```python
from build123d import *

# Parameters (mm, degrees)
F0_R     = 2.38125
F0_R_2   = 1.143
F1_DEPTH = 4.7625
F2_R     = 6.35
F3_DEPTH = 7.62
F4_DEPTH = 5.08


with BuildPart() as f1:
    # F0 (on Top) → F1 (new body)
    with BuildSketch(Plane.XY):
        with BuildLine():
            Line((21.5265, 64.595826), (21.5265, 76.2))
            Line((21.5265, 76.2), (14.2875, 76.2))
            Line((14.2875, 76.2), (14.2875, 72.5805))
            ThreePointArc((14.2875, 72.5805), (0, 58.293), (-14.2875, 72.5805))
            Line((-14.2875, 72.5805), (-14.2875, 76.2))
            Line((-14.2875, 76.2), (-21.5265, 76.2))
            Line((-21.5265, 76.2), (-21.5265, 64.595826))
            Line((-21.5265, 64.595826), (-11.1125, 52.489269))
            Line((-11.1125, 52.489269), (-11.1125, -76.2))
            Line((-11.1125, -76.2), (11.1125, -76.2))
            Line((11.1125, -76.2), (11.1125, 52.489269))
            Line((11.1125, 52.489269), (21.5265, 64.595826))
        make_face()
        with Locations((-17.907, 72.5805)):
            Circle(F0_R, mode=Mode.SUBTRACT)
        with Locations((17.907, 72.5805)):
            Circle(F0_R, mode=Mode.SUBTRACT)
        with Locations((-17.907, 72.5805)):
            Circle(F0_R)
        with Locations((-17.907, 72.5805)):
            Circle(F0_R_2, mode=Mode.SUBTRACT)
        with Locations((17.907, 72.5805)):
            Circle(F0_R)
        with Locations((17.907, 72.5805)):
            Circle(F0_R_2, mode=Mode.SUBTRACT)
        with Locations((-17.907, 72.5805)):
            Circle(F0_R_2)
        with Locations((17.907, 72.5805)):
            Circle(F0_R_2)
    extrude(amount=-F1_DEPTH)

    # F2
    f2_edges = [f1.edges().sort_by_distance(p)[0] for p in [
        (21.5265, 64.595826, -2.38125),
        (11.1125, 52.489269, -2.38125),
        (-21.5265, 64.595826, -2.38125),
        (-11.1125, 52.489269, -2.38125),
    ]]
    fillet(f2_edges, radius=F2_R)

    # F0 (on Top) → F3 (join)
    with BuildSketch(Plane.XY):
        with Locations((17.907, 72.5805)):
            Circle(F0_R_2)
        with Locations((-17.907, 72.5805)):
            Circle(F0_R_2)
    extrude(amount=F3_DEPTH)

    # F0 (on Top) → F4 (join)
    with BuildSketch(Plane.XY):
        with Locations((-17.907, 72.5805)):
            Circle(F0_R)
        with Locations((-17.907, 72.5805)):
            Circle(F0_R_2, mode=Mode.SUBTRACT)
        with Locations((17.907, 72.5805)):
            Circle(F0_R)
        with Locations((17.907, 72.5805)):
            Circle(F0_R_2, mode=Mode.SUBTRACT)
    extrude(amount=F4_DEPTH)


solid = f1.part
```
Can you work these out from the model? Positions are in its coordinate system, mm. A direction names the side the tool comes from. Give positions to 0.01 mm unless a question says otherwise; leave off trailing zeros. Loops run counter-clockwise (first coordinate to the right, second up) from the corner with the lowest first, then second, coordinate; pieces in that order, holes last. Notation, with made-up numbers: M 71,-37.5 L 99,-37.5 A29 ccw 99,-11.5 Z; hole C 64,5.5 d9. An arc over 180 degrees is marked long. One line per question, with ' | ' between items. Start each with the question number.
Q1. If we section it at B-B (x = 0): Please give me the cut outline in (y, z).
Q2. For faces 1 (the flat face through (-14.288, 74, -2)), 2 (the cylindrical face through (-18.423, 70.256, 2.504)), 3 (the flat face through (21.526, 72, -2)), 4 (the flat face through (11.112, -14, -2)), 5 (the flat face through (0, -76.2, -2)), which set-ups out of +Z, -Z, +X, -X, +Y, -Y let a thin tool reach every point of the face, with its end or its side?
Q3. For pin 1 Ø1.4 at (y, z) = (-32.5, -3.5) entering from +X; pin 2 Ø4 at (x, z) = (-17, 2.5) entering from -Y; pin 3 Ø1.4 at (y, z) = (-14, -3.5) entering from -X, each with a flat end and sliding along its axis, tell me the tip position at first contact or that it passes through.
Q4. If we section it at C-C (y = -52.5): Please give me the cut outline in (x, z).
Q5. If we mould it in two halves opening along X, with no side actions, what happens to faces 6 (the flat face through (18, 76.2, -2)), 7 (the flat face through (18, 74, 5.08)), 8 (the cylindrical face through (21.14, 64.77, -2.41)), 9 (the cylindrical face through (-21.14, 64.77, -2.41))? For each: +X half, -X half, draft (parallel to the pull), parting line (faces both ways), or undercut.
Q6. If I drill on line 1 (X direction, y = -9.5, z = -2.75); line 2 (Z direction, x = -3, y = -23.5); line 3 (Y direction, x = -7.5, z = -0.25), over which ranges is the centre line in solid material (lowest first)? Write a range as from..to.
Computed:
1) outline: M -76.2,-4.76 L 58.29,-4.76 L 58.29,0 L -76.2,0 Z
2) face 1: +Z, -Z, +Y | face 2: +Z | face 3: +Z, -Z, +X, +Y, -Y | face 4: +Z, -Z, +X, -Y | face 5: +Z, -Z, +X, -X, -Y
3) pin 1: stops at x = 11.11 | pin 2: stops at y = 70.2 | pin 3: stops at x = -11.11
4) outline: M -11.11,-4.76 L 11.11,-4.76 L 11.11,0 L -11.11,0 Z
5) face 6: draft | face 7: undercut | face 8: +X half | face 9: -X half
6) line 1: x = -11.11..11.11 | line 2: z = -4.76..0 | line 3: y = -76.2..60.42
